Check sheet for the modelled part. Datum: model origin and axes. Units: mm. A direction names the side the tool comes from. Give positions to 0.01 mm unless a question says otherwise; leave off trailing zeros. Loops run counter-clockwise (first coordinate to the right, second up) from the corner with the lowest first, then second, coordinate; pieces in that order, holes last. Notation, with made-up numbers: (2, -20) -> (10, -20) arc R10 cw to (10, -2) -> close; hole circle Ø6 at (36, 17). An arc over 180 degrees is marked (long way). Write each question's results on one line, items separated by ' | '. Start each with the question number.
Item 1: Mould release check, pull along X, two halves, no side actions. Record for faces 1 (the face through (0.439, -0.746, 0.493)), 2 (the face through (0, 0, 28)), 3 (the face through (-0.54, -2.44, 2.96)): pulls with the +X half, pulls with the -X half, needs draft (parallel to the pull), parting line crosses it, or undercut.
Item 2: Cross-section at A-A on y = 0. Enter the section's corners in (x, z), then the cut area to 3 significant figures.
Item 3: Access from +Z, -Z, +X, -X, +Y, -Y to the whole of each face (thin tool, end or side, straight path). Record for faces 4 (the face through (0.866, 0, 0.5)), 5 (the face through (1.1, 0, 0)), 6 (the face through (-1.5, 0.07, 17.1)).
Item 4: Scan lines: line 1 along Z through (x, y) = (-0.1, -0.35); line 2 along Z through (x, y) = (-1.8, -1.25); line 3 along X through (y, z) = (-1.15, 24). Record each from-to range of solid material in increasing order.
Item 5: Cross-section at B-B on z = 16. Enter the section's corners in (x, y), then the cut area to 3 significant figures.
from build123d import *

# Parameters (mm, degrees)
SKETCH1_R           = 2.5
BOSS_EXTRUDE1_DEPTH = 6
SKETCH2_R           = 1.5
BOSS_EXTRUDE2_DEPTH = 22
CUT_EXTRUDE1_DEPTH  = 1
CHAMFER1_SIZE       = 0.5


with BuildPart() as part:
    # Sketch1 → Boss-Extrude1 (new body)
    with BuildSketch(Plane.XY):
        Circle(SKETCH1_R)
    extrude(amount=BOSS_EXTRUDE1_DEPTH)

    # Sketch2 → Boss-Extrude2 (add)
    with BuildSketch(Plane.XY.offset(6)):
        Circle(SKETCH2_R)
    extrude(amount=BOSS_EXTRUDE2_DEPTH)

    # Sketch3 → Cut-Extrude1 (cut)
    with BuildSketch(Plane(origin=(0, 0, 0), x_dir=(-1, 0, 0), z_dir=(0, 0, -1))):
        Polygon((0, 1), (-0.866025404, 0.5), (-0.866025404, -0.5), (0, -1), (0.866025404, -0.5), (0.866025404, 0.5), align=None)
    extrude(amount=-CUT_EXTRUDE1_DEPTH, mode=Mode.SUBTRACT)

    # Chamfer1
    chamfer1_edges = [part.edges().sort_by_distance(p)[0] for p in [
        (-1.5, 0, 6),
    ]]
    chamfer(chamfer1_edges, length=CHAMFER1_SIZE)


solid = part.part
Answer sheet:
1) face 1: undercut | face 2: needs draft | face 3: parting line crosses it
2) outline: (-2.5, 0) -> (-0.87, 0) -> (-0.87, 1) -> (0.87, 1) -> (0.87, 0) -> (2.5, 0) -> (2.5, 6) -> (2, 6) -> (1.5, 6.5) -> (1.5, 28) -> (-1.5, 28) -> (-1.5, 6.5) -> (-2, 6) -> (-2.5, 6) -> close | area: 94.5 mm²
3) face 4: -Z | face 5: -Z, +X, -X, +Y, -Y | face 6: +Z
4) line 1: z = 1 to 28 | line 2: z = 0 to 6 | line 3: x = -0.96 to 0.96
5) outline: circle Ø3 at (0, 0) | area: 7.07 mm²
